from build123d import *

# Parameters (mm, degrees)
BASPROSKE_W              = 5
BASPROSKE_H              = 18
TOOTHCUT_DEPTH           = 26.942243542
TEETHCUTS_COUNT          = 16
TEETHCUTS_ANGLE          = 337.5
BORSKE_R                 = 2.5
BORE_DEPTH               = 50.0000508
BOSS_EXTRUDE1_DEPTH      = 7
BOSS_EXTRUDE1_DEPTH_BACK = 5
SKETCH1_R                = 10
SKETCH2_R                = 1.25
BOSS_EXTRUDE3_DEPTH      = 1.8
BOSS_EXTRUDE4_DEPTH      = 10
FILLET1_R                = 2


with BuildPart() as part:
    # BasProSke → Base-Revolve (revolve)
    with BuildSketch(Plane(origin=(0, 0, 0), x_dir=(1, 0, 0), z_dir=(0, 1, 0)), mode=Mode.PRIVATE) as base_revolve_sk:
        with Locations((2.5, 9)):
            Rectangle(BASPROSKE_W, BASPROSKE_H)
    revolve(base_revolve_sk.sketch.rotate(Axis((-10, 0, 0), (1, 0, 0)), 180), axis=Axis((-10, 0, 0), (1, 0, 0)))

    # TooCutSke → ToothCut (cut, through all)
    with BuildSketch(Plane(origin=(0, 0, 0), x_dir=(0, 0, -1), z_dir=(1, 0, 0))):
        with BuildLine():
            ThreePointArc((1.03434411, 13.459313997), (0, 13.499), (-1.03434411, 13.459313997))
            ThreePointArc((-1.03434411, 13.459313997), (-1.635143665, 15.806872195), (-3.065655864, 17.762792553))
            ThreePointArc((-3.065655864, 17.762792553), (0, 18.0254), (3.065655864, 17.762792553))
            ThreePointArc((3.065655864, 17.762792553), (1.635143665, 15.806872195), (1.03434411, 13.459313997))
        make_face()
    toothcut = extrude(amount=TOOTHCUT_DEPTH, mode=Mode.SUBTRACT)

    # TeethCuts: ToothCut ×16 about axis
    teethcuts_axis = Axis((-10, 0, 0), (1, 0, 0))
    for i in range(1, TEETHCUTS_COUNT):
        add(toothcut.rotate(teethcuts_axis, i * TEETHCUTS_ANGLE / (TEETHCUTS_COUNT - 1)), mode=Mode.SUBTRACT)

    # BorSke → Bore (cut, symmetric)
    with BuildSketch(Plane(origin=(0, 0, 0), x_dir=(0, 0, -1), z_dir=(1, 0, 0))):
        with Locations(Location((0, 0, 0), (0, 0, 180))):
            Circle(BORSKE_R)
    extrude(amount=BORE_DEPTH, both=True, mode=Mode.SUBTRACT)

    # Sketch1 → Boss-Extrude1 (add, two sides: drawn at the far end of the back side and taken through both)
    with BuildSketch(Plane.ZY.offset(-BOSS_EXTRUDE1_DEPTH_BACK)):
        Circle(SKETCH1_R)
    extrude(amount=BOSS_EXTRUDE1_DEPTH + BOSS_EXTRUDE1_DEPTH_BACK)

    # Sketch2 → Boss-Extrude3 (add)
    with BuildSketch(Plane.ZY.offset(7)):
        with Locations((-9.092660354, 4.162154213)):
            Circle(SKETCH2_R)
    extrude(amount=-BOSS_EXTRUDE3_DEPTH)

    # Sketch3 → Boss-Extrude4 (add)
    with BuildSketch(Plane(origin=(5, 0, 0), x_dir=(0, 0, -1), z_dir=(1, 0, 0))):
        with BuildLine():
            Line((2.5, 7), (2.5, -7))
            ThreePointArc((2.5, -7), (0, -9.5), (-2.5, -7))
            Line((-2.5, -7), (-2.5, 7))
            ThreePointArc((-2.5, 7), (0, 9.5), (2.5, 7))
        make_face()
    extrude(amount=BOSS_EXTRUDE4_DEPTH)

    # Fillet1
    fillet1_edges = [part.edges().sort_by_distance(p)[0] for p in [
        (5, 9.5, 0),
        (5, 0, 2.5),
        (5, -9.5, 0),
        (5, 0, -2.5),
    ]]
    fillet(fillet1_edges, radius=FILLET1_R)


solid = part.part
Verification items for the finished model (mm, model axes). A direction names the side the tool comes from. Give positions to 0.01 mm unless a question says otherwise; leave off trailing zeros. Order: outer loops, then holes, each group sorted by start corner. A loop starts at its lowest first (then second) coordinate and runs counter-clockwise, first axis right, second up. Notation, with made-up numbers: M 35.5,76 L 85.5,76 A23 ccw 85.5,110 Z; hole C 59.5,-35.5 d10. An arc over 180 degrees is marked long. Answer as a JSON object with one key per item and string values. Group by question number.
1) Cross-section at C-C (x = 6.25). Enter the section's corners in (y, z).
2) Mould release check, pull along Y, two halves, no side actions. Record for faces 1 (the face through (2.535, 17.655, 3.505)), 2 (the face through (5, 0, 8)), 3 (the face through (2.465, -12.466, 5.179)): released by +Y, released by -Y, zero draft, split by the parting line, or undercut.
3) Scan lines: line 1 along X through (y, z) = (-12, 0); line 2 along Y through (x, z) = (4.75, 8.5); line 3 along Z through (x, y) = (-1.5, -4). Record each from-to range of solid material in increasing order. Write a range as [from, to].
4) Cross-section at D-D (z = -11.5). Enter the section's corners in (x, y), then the cut area to 3 significant figures.
5) Access from +Z, -Z, +X, -X, +Y, -Y to the whole of each face (thin tool, end or side, straight path). Record for faces 4 (the face through (2.465, 1.614, -15.762)), 5 (the face through (11, 0, -2.5)), 6 (the face through (-5.2, 4, -10)), 7 (the face through (2.465, 13.99, -7.573)), 8 (the face through (2.465, 4.537, -15.247)).
6) Cross-section at A-A (z = 0). Enter the section's corners in (x, y).
7) Depth check by flat-ended pin: pin 1 Ø2.5 at (x, y) = (12.5, 1.5) entering from -Z; pin 2 Ø5 at (x, z) = (6, -8.5) entering from +Y; pin 3 Ø9 at (x, y) = (11, -1) entering from +Z. Enter the tip coordinate at first touch or a pass-through.
8) Cross-section at B-B (y = 0). Enter the section's corners in (x, z).
Result sheet:
{
 "1": {"outline": "M -7,-2.65 L 7,-2.65 A2.65 ccw 7,2.65 L -7,2.65 A2.65 ccw Z"},
 "2": {"face 1": "released by +Y", "face 2": "zero draft", "face 3": "undercut"},
 "3": {"line 1": "x = [0, 5]", "line 2": "y = [-14.69, 14.69]", "line 3": "z = [-9.17, 9.17]"},
 "4": {"outline": "M 0,-9.65 L 5,-9.65 L 5,9.65 L 0,9.65 Z", "area": "96.5 mm2"},
 "5": {"face 4": "-Z, +X, -X", "face 5": "-Z, +X, +Y, -Y", "face 6": "-Z, +Y", "face 7": "+X, -X, +Y", "face 8": "+X, -X"},
 "6": {"outline": "M -7,-10 L 0,-10 L 0,-13.5 L 5,-13.5 L 5,-11.5 A2 cw 7,-9.5 L 15,-9.5 L 15,9.5 L 7,9.5 A2 cw 5,11.5 L 5,13.5 L 0,13.5 L 0,10 L -7,10 Z"},
 "7": {"pin 1": "stops at z = -2.5", "pin 2": "stops at y = 15.23", "pin 3": "stops at z = 2.56"},
 "8": {"outline": "M -7,-10 L 0,-10 L 0,-13.5 L 5,-13.5 L 5,-4.5 A2 cw 7,-2.5 L 15,-2.5 L 15,2.5 L 7,2.5 A2 cw 5,4.5 L 5,13.5 L 0,13.5 L 0,10 L -7,10 Z"}
}
